Check sheet for the modelled part. Datum: model origin and axes. Units: mm. A direction names the side the tool comes from. Round coordinates to 2 decimals unless told otherwise and drop trailing zeros. Order: outer loops, then holes, each group sorted by start corner. A loop starts at its lowest first (then second) coordinate and runs counter-clockwise, first axis right, second up. Notation, with made-up numbers: (55, 30.5) -> (61, 30.5) arc R14 ccw to (61, 53.5) -> close; hole circle Ø2 at (-14.75, 23). An arc over 180 degrees is marked (long way). Use CSV: the item, a comma, the result in double quotes.
Autodesk Inventor part; units mm, degrees
ref_plane "YZ Plane" through (0, 0, 0) normal (1, 0, 0) x (0, 1, 0)
ref_plane "XZ Plane" through (0, 0, 0) normal (0, 1, 0) x (-1, 0, 0)
ref_plane "XY Plane" through (0, 0, 0) normal (0, 0, 1) x (1, 0, 0)
ref_plane "Work Plane1" through (0, 0, 0) normal (0, 0, 1) x (1, 0, 0)
sketch "Sketch2" plane through (0, 0, 0) normal (0, 0, 1) x (1, 0, 0)
  line L0 (-69.85, 121.9708) -> (69.85, 121.9708)
  line L1 (-69.85, 33.0708) -> (-69.85, 121.9708)
  line L2 (69.85, 33.0708) -> (-69.85, 33.0708)
  line L3 (-50.8, 64.8208) -> (-50.8, 33.0708)
  line L4 (50.8, 64.8208) -> (-50.8, 64.8208)
  line L5 (50.8, 33.0708) -> (50.8, 64.8208)
  line L6 (69.85, 121.9708) -> (69.85, 33.0708)
  line L7 (-15.2718, 85.3756) -> (-15.2718, 64.8208)
  line L8 (15.24, 85.3756) -> (-15.2718, 85.3756)
  line L9 (15.24, 64.8208) -> (15.24, 85.3756)
  point P0 (0, 0)
extrude "Extrusion1" add sketch "Sketch2" along normal blind 6.35 contours L0 L6 L2 L5 L4 L9 L8 L7 L3 L1
sketch "Sketch3" plane through (0, 0, 6.35) normal (0, 0, 1) x (1, 0, 0)
  circle A0 centre (-57.15, 45.7708) radius 3.5662
  circle A1 centre (-25.4, 73.7616) radius 2.4892
  circle A2 centre (57.15, 45.7708) radius 3.9624
  point P0 (0, 0)
  point P1 (25.4, 73.7616)
  point P2 (25.4, 73.7616)
hole "Hole1" at (25.4, 73.7616, 6.35) at (-57.15, 45.7708, 6.35) at (57.15, 45.7708, 6.35) at (-25.4, 73.7616, 6.35) direction (0, 0, -1) diameter 6.35 depth 25.4 tip angle 118
sketch "Sketch5" plane through (0, 0, 6.35) normal (0, 0, 1) x (1, 0, 0)
  line L0 (-69.85, 33.0708) -> (-50.8, 33.0708)
  line L1 (-69.85, 33.0708) -> (-82.55, 33.0708)
  line L2 (-82.55, 33.0708) -> (-82.55, 134.6708)
  line L3 (-82.55, 134.6708) -> (-69.85, 134.6708)
  line L4 (-69.85, 134.6708) -> (-69.85, 33.0708)
  line L5 (-82.55, 134.6708) -> (82.55, 134.6708)
  line L6 (82.55, 134.6708) -> (82.55, 121.9708)
  line L7 (82.55, 121.9708) -> (-82.55, 121.9708)
  line L8 (-82.55, 121.9708) -> (-82.55, 134.6708)
  line L9 (50.8, 33.0708) -> (69.85, 33.0708)
  line L10 (82.55, 121.9708) -> (69.85, 121.9708)
  line L11 (69.85, 121.9708) -> (69.85, 33.0708)
  line L12 (69.85, 33.0708) -> (82.55, 33.0708)
  line L13 (82.55, 33.0708) -> (82.55, 121.9708)
  point P0 (0, 0)
  dimension "d26" = 12.7
  dimension "d27" = 12.7
  dimension "d28" = 12.7
extrude "Extrusion3" add sketch "Sketch5" against normal up to surface (6.35 mm away)
ref_plane "Work Plane2" through (0, 33.0708, 6.35) normal (-1, 0, 0) x (0, 0, 1)
equation "\"d1\" = d2"
properties part number "Hang Mount"
Q1. Sectioned sample at B-B, the plane z = 3. Enter the section's corners in (x, y) (3 decimals).
Result sheet:
outline,"(-82.55, 33.071) -> (-50.8, 33.071) -> (-50.8, 64.821) -> (-15.272, 64.821) -> (-15.272, 85.376) -> (15.24, 85.376) -> (15.24, 64.821) -> (50.8, 64.821) -> (50.8, 33.071) -> (82.55, 33.071) -> (82.55, 134.671) -> (-82.55, 134.671) -> close; hole circle Ø6.35 at (-57.15, 45.771); hole circle Ø6.35 at (-25.4, 73.762); hole circle Ø6.35 at (25.4, 73.762); hole circle Ø6.35 at (57.15, 45.771)"
Q2. Scan lines: L1, parallel to Y at x = -57.15, z = 4.5; L2, parallel to Y at x = 25.4, z = 2.75; L3, parallel to X at y = 78.5, z = 5.5. Record each from-to range of solid material in increasing order.
Result sheet:
L1,"y = 33.07 to 42.6, 48.95 to 134.67"
L2,"y = 64.82 to 70.59, 76.94 to 134.67"
L3,"x = -82.55 to -15.27, 15.24 to 82.55"
Q3. Mould release check, pull along Y, two halves, no side actions. Record for faces 3 (the face through (-26.35, 70.73, 3.13)), 4 (the face through (-50.8, 49, 3)), 5 (the face through (-1, 134.671, 3)): pulls with the +Y half, pulls with the -Y half, needs draft (parallel to the pull), parting line crosses it, or undercut.
Result sheet:
face 3,"undercut"
face 4,"needs draft"
face 5,"pulls with the +Y half"
Q4. Sectioned sample at C-C, the plane x = -57.15. Enter the section's corners in (y, z), then the cut area to 3 significant figures.
Result sheet:
outline,"(33.07, 0) -> (42.6, 0) -> (42.6, 6.35) -> (33.07, 6.35) -> close; (48.95, 0) -> (134.67, 0) -> (134.67, 6.35) -> (48.95, 6.35) -> close"
area,"605 mm^2"
Q5. Sectioned sample at D-D, the plane x = 3.5. Enter the section's corners in (y, z), then the cut area to 3 significant figures.
Result sheet:
outline,"(85.38, 0) -> (134.67, 0) -> (134.67, 6.35) -> (85.38, 6.35) -> close"
area,"313 mm^2"
Q6. Access from +Z, -Z, +X, -X, +Y, -Y to the whole of each face (thin tool, end or side, straight path). Record for faces 1 (the face through (67, 33.071, 3)), 2 (the face through (50.8, 49, 3)).
Result sheet:
face 1,"+Z, -Z, +X, -X, -Y"
face 2,"+Z, -Z, -Y"
Q7. Sectioned sample at A-A, the plane y = 81. Enter the section's corners in (x, z), then the cut area to 3 significant figures.
Result sheet:
outline,"(-82.55, 0) -> (-15.27, 0) -> (-15.27, 6.35) -> (-82.55, 6.35) -> close; (15.24, 0) -> (82.55, 0) -> (82.55, 6.35) -> (15.24, 6.35) -> close"
area,"855 mm^2"
Q8. Go/stop test with flat-tipped pins: pin 1 (3 mm diameter, centred on x = 13, z = 4.5, fed in from -Y); pin 2 (1.9 mm diameter, centred on x = 36.5, z = 4, fed in from -Y). Record where each tip stops, or that it passes through.
Result sheet:
pin 1,"stops at y = 85.38"
pin 2,"stops at y = 64.82"
